```python
from build123d import *

# Parameters (mm, degrees)
SKETCH1_R           = 2.5
BOSS_EXTRUDE1_DEPTH = 3


with BuildPart() as part:
    # Sketch1 → Boss-Extrude1 (new body)
    with BuildSketch(Plane.XY):
        with BuildLine():
            Line((0, 10), (0, 0))
            Line((0, 0), (15, 0))
            Line((15, 0), (15, 3))
            Line((15, 3), (39.8, 3))
            Line((39.8, 3), (39.8, 0))
            Line((39.8, 0), (60.2, 0))
            Line((60.2, 0), (60.2, 3))
            Line((60.2, 3), (85, 3))
            Line((85, 3), (85, 0))
            Line((85, 0), (100, 0))
            Line((100, 0), (100, 10))
            Line((100, 10), (97, 10))
            Line((97, 10), (97, 29.8))
            Line((97, 29.8), (100, 29.8))
            Line((100, 29.8), (100, 100))
            ThreePointArc((100, 100), (50, 150), (0, 100))
            Line((0, 100), (0, 29.8))
            Line((0, 29.8), (3, 29.8))
            Line((3, 29.8), (3, 10))
            Line((3, 10), (0, 10))
        make_face()
        with Locations((50, 100)):
            Circle(SKETCH1_R, mode=Mode.SUBTRACT)
    extrude(amount=BOSS_EXTRUDE1_DEPTH)


solid = part.part
```
Input: part model. Units: mm. Frame: model coordinates. A direction names the side the tool comes from. Give positions to 0.01 mm unless a question says otherwise; leave off trailing zeros. Order: outer loops, then holes, each group sorted by start corner. A loop starts at its lowest first (then second) coordinate and runs counter-clockwise, first axis right, second up. Notation, with made-up numbers: M -35,12.25 L -1,12.25 A18 ccw -1,45.25 Z; hole C 71,-26.75 d11. An arc over 180 degrees is marked long. Return JSON: item names as keys, results as strings.
1) Section query D-D on x = 92. Output: boundary loops of the cut face in (y, z), and give its area (3 significant figures).
Taken from the geometry:
{"outline": "M 0,0 L 127.13,0 L 127.13,3 L 0,3 Z", "area": "381 mm2"}
2) Section query A-A on x = 50. Output: boundary loops of the cut face in (y, z), and give its area (3 significant figures).
Taken from the geometry:
{"outline": "M 0,0 L 97.5,0 L 97.5,3 L 0,3 Z; M 102.5,0 L 150,0 L 150,3 L 102.5,3 Z", "area": "435 mm2"}
3) Section query B-B on z = 2.15. Output: boundary loops of the cut face in (x, y), and give its area (3 significant figures).
Taken from the geometry:
{"outline": "M 0,0 L 15,0 L 15,3 L 39.8,3 L 39.8,0 L 60.2,0 L 60.2,3 L 85,3 L 85,0 L 100,0 L 100,10 L 97,10 L 97,29.8 L 100,29.8 L 100,100 A50 ccw 0,100 L 0,29.8 L 3,29.8 L 3,10 L 0,10 Z; hole C 50,100 d5", "area": "13,600 mm2"}
4) Line query: L1, parallel to Y at x = 50, z = 2.1; L2, parallel to Y at x = 26, z = 2.45; L3, parallel to Y at x = 37, z = 0.6. Output: solid intervals per line, ascending. Write a range as [from, to].
Taken from the geometry:
{"L1": "y = [0, 97.5], [102.5, 150]", "L2": "y = [3, 143.86]", "L3": "y = [3, 148.28]"}
5) Contact query for flat-ended pins moving along their axis: pin 1 (1 mm diameter, centred on y = 116.5, z = 2, fed in from +X); pin 2 (1.5 mm diameter, centred on y = 128, z = 2, fed in from +X); pin 3 (3 mm diameter, centred on x = 50, y = 100, fed in from -Z); pin 4 (0.9 mm diameter, centred on y = 15, z = 2, fed in from +X). Output: stop coordinate, or through.
Taken from the geometry:
{"pin 1": "stops at x = 97.37", "pin 2": "stops at x = 91.92", "pin 3": "passes through", "pin 4": "stops at x = 97"}
6) Access query for faces 1 (the face through (97, 20, 1)), 2 (the face through (7, 0, 1)), 3 (the face through (51.099, 149.988, 1.479)), 4 (the face through (1, 29.8, 1)), 5 (the face through (15, 1, 1)). Directions: +Z, -Z, +X, -X, +Y, -Y. A direction counts if a zero-diameter tool reaches every point of the face in a straight line with its end or side. Return the directions, or none.
Taken from the geometry:
{"face 1": "+Z, -Z, +X", "face 2": "+Z, -Z, +X, -X, -Y", "face 3": "+Z, -Z, +Y", "face 4": "+Z, -Z, -X", "face 5": "+Z, -Z, -Y"}
7) Mould query, pull axis X, two halves, no side actions, for faces 6 (the face through (98, 29.8, 1)), 7 (the face through (0, 65, 1)), 8 (the face through (85, 2, 1)). Classes: released by +X, released by -X, zero draft, split by the parting line, or undercut.
Taken from the geometry:
{"face 6": "zero draft", "face 7": "released by -X", "face 8": "undercut"}
8) Section query C-C on y = 126. Output: boundary loops of the cut face in (x, z).
Taken from the geometry:
{"outline": "M 7.29,0 L 92.71,0 L 92.71,3 L 7.29,3 Z"}
